Can you work these out from the model? Positions are in its coordinate system, mm. Round coordinates to 2 decimals unless told otherwise and drop trailing zeros. Write each loop counter-clockwise with the first axis right and the second up, starting at its lowest first coordinate (ties: lowest second). Pieces come first, ordered by that corner, then holes. Notation, with made-up numbers: M 44,-34.75 L 103,-34.75 A18 ccw 103,-2.75 Z; hole C 18.5,75.5 d4. An arc over 180 degrees is marked long. Answer in a Markdown table with one row per item. Add a question column.
(1) I'm going to push flat-ended pins straight in: pin 1 (10 mm diameter, centred on x = 825.5, z = 33.5, fed in from -Y); pin 2 (8 mm diameter, centred on x = 700.5, z = 22, fed in from -Y); pin 3 (5 mm diameter, centred on x = 281.5, z = 31, fed in from +Y). Where does each tip first touch, or does it pass through?
(2) Suppose I cut it at C-C, the plane x = 172.5. Write out the boundary of the cut face in (y, z), then the cut area to 3 significant figures.
(3) If I drill on probe 1 along Y at (x, z) = (0, 12); probe 2 along X at (y, z) = (1388.5, 37); probe 3 along X at (y, z) = (1323, 35), over which ranges is the centre line in solid material (lowest first)?
from build123d import *

# Parameters (mm, degrees)
F0_R     = 5
F1_DEPTH = 50


with BuildPart() as f1:
    # F0 (on Top) → F1 (new body)
    with BuildSketch(Plane.XY):
        with BuildLine():
            Line((0, 1505.000002), (0, 1500.009527))
            ThreePointArc((0, 1500.009527), (4.982806, 1501.339369), (8.640344, 1504.975199))
            ThreePointArc((8.640344, 1504.975199), (4.32019, 1504.993801), (0, 1505.000002))
        make_face()
        with BuildLine():
            ThreePointArc((10, 1510.009527), (-7.071068, 1517.080595), (0, 1500.009527))
            Line((0, 1500.009527), (0, 1505.000002))
            ThreePointArc((0, 1505.000002), (4.32019, 1504.993801), (8.640344, 1504.975199))
            ThreePointArc((8.640344, 1504.975199), (9.654104, 1507.402176), (10, 1510.009527))
        make_face()
        with Locations((0, 1510.009527)):
            Circle(F0_R, mode=Mode.SUBTRACT)
        with BuildLine():
            ThreePointArc((0, 1500), (535.233135, 1401.258538), (1000, 1118.033989))
            Line((1000, 1118.033989), (1003.333335, 1121.76077))
            ThreePointArc((1003.333335, 1121.76077), (541.050835, 1404.38207), (8.640344, 1504.975199))
            ThreePointArc((8.640344, 1504.975199), (4.982806, 1501.339369), (0, 1500.009527))
            Line((0, 1500.009527), (0, 1500))
        make_face()
    extrude(amount=F1_DEPTH)


solid = f1.part
Calculated:
| question | item | result |
|---|---|---|
| 1 | pin 1 | y = 1249.11 |
| 1 | pin 2 | y = 1324.27 |
| 1 | pin 3 | y = 1478.91 |
| 2 | outline | M 1490.05,0 L 1495.08,0 L 1495.08,50 L 1490.05,50 Z |
| 2 | area | 252 mm² |
| 3 | probe 1 | 1500.01 to 1505.01, 1515.01 to 1520.01 |
| 3 | probe 2 | 567.51 to 580.6 |
| 3 | probe 3 | 706.87 to 717.42 |
